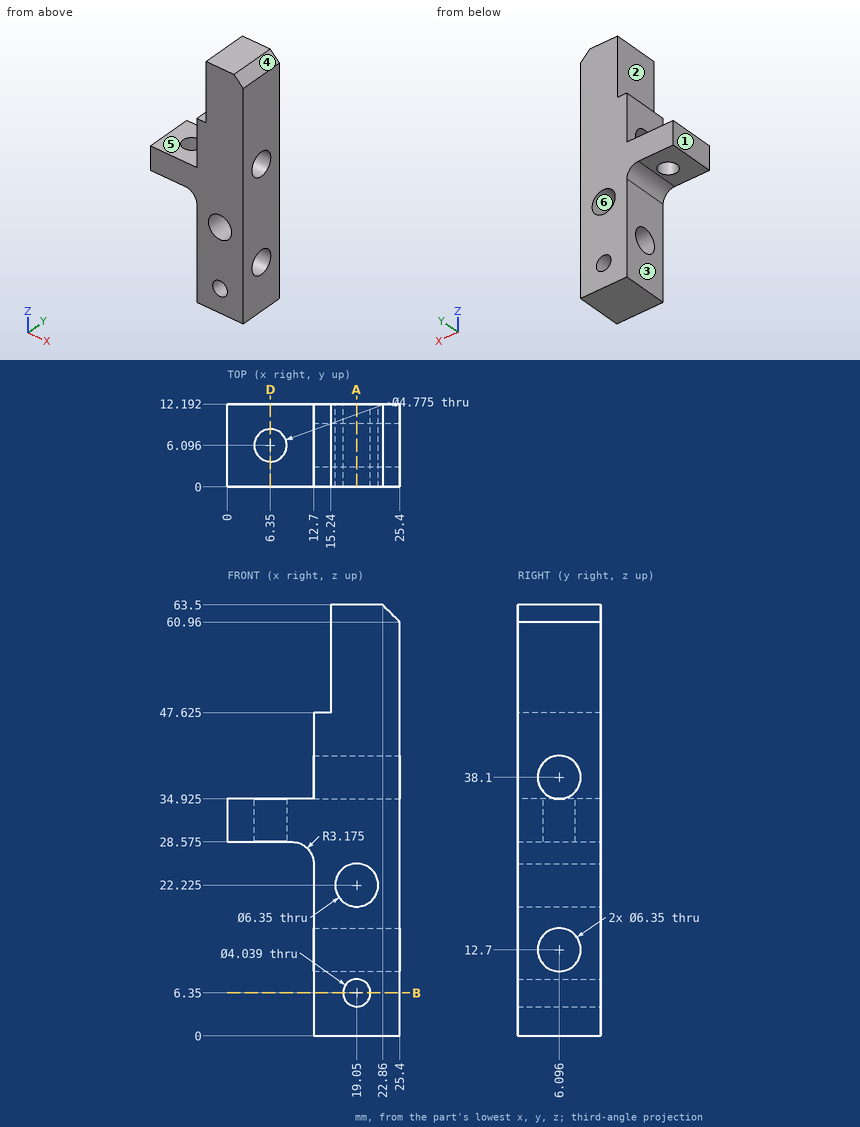
Study the drawing (mm; zero at the part's minimum x, y, z) and answer. A direction names the side the tool comes from. Give positions to 0.01 mm unless a question says otherwise; leave off trailing zeros. Order: outer loops, then holes, each group sorted by start corner. A loop starts at its lowest first (then second) coordinate and runs counter-clockwise, first axis right, second up. Notation, with made-up numbers: (51.5, -34) -> (96.5, -34) arc R26 ccw to (96.5, 5) -> close; hole circle Ø10 at (35, -20.75). An arc over 180 degrees is marked (long way). Put each result on its own line as item: value.
Item 1: For the marked faces 1, 2 and 3, determine the directions among +Z, -Z, +X, -X, +Y, -Y from which every point of the face is accessible in a straight line to the end or side of a thin tool.
Established:
face 1: +Z, -Z, -X, +Y, -Y
face 2: +Z, -X, +Y, -Y
face 3: -Z, -X, +Y, -Y
Item 2: A cutting plane is placed at D-D on x = 6.35. Give the vertices of the cut face in (y, z) (1 decimal), plus the area to 3 significant figures.
Established:
outline: (0, 28.6) -> (3.7, 28.6) -> (3.7, 34.9) -> (0, 34.9) -> close; (8.5, 28.6) -> (12.2, 28.6) -> (12.2, 34.9) -> (8.5, 34.9) -> close
area: 47.1 mm^2
Item 3: For a pull along X with two mould halves and no side action, classify the marked faces 4, 5 and 6 as released by +X, released by -X, zero draft, split by the parting line, or undercut.
Established:
face 4: released by +X
face 5: zero draft
face 6: undercut
Item 4: Given P1, Ø5, axis at x = 8, y = 8, coming from the -Z side; P2, Ø5.5, axis at x = 6.35, y = 6.096, coming from the +Z side (3 decimals); P3, Ø2, axis at x = 13.5, y = 8, coming from the +Z side (3 decimals); P4, Ø4, axis at y = 6.096, z = 12.7, coming from the -X side, each flat-ended and moving along its own axis, determine where each tip first touches the part or whether it passes through.
Established:
P1: stops at z = 28.42
P2: stops at z = 34.925
P3: stops at z = 47.625
P4: passes through
Item 5: Straight lines are drawn through the part: line 1 (Z direction, x = 19, y = 2.5); line 2 (Y direction, x = 6.35, z = 33.5); line 3 (Z direction, x = 19.05, y = 7.75). For each, find the intervals that lie inside material, in ascending order.
Established:
line 1: z = 0 to 4.33, 8.37 to 19.05, 25.4 to 63.5
line 2: y = 0 to 3.71, 8.48 to 12.19
line 3: z = 0 to 4.33, 8.37 to 9.99, 15.41 to 19.05, 25.4 to 35.39, 40.81 to 63.5
Item 6: A cutting plane is placed at B-B on z = 6.35. Give the vertices of the cut face in (x, y), plus the area to 3 significant figures.
Established:
outline: (12.7, 0) -> (17.03, 0) -> (17.03, 12.19) -> (12.7, 12.19) -> close; (21.07, 0) -> (25.4, 0) -> (25.4, 12.19) -> (21.07, 12.19) -> close
area: 106 mm^2
Item 7: A cutting plane is placed at A-A on x = 19.05. Count the separate pieces of the cut face and the enclosed holes in it, plus the area to 3 significant figures.
Established:
separate pieces: 3
enclosed holes: 2
area: 584 mm^2
